from build123d import *

# Parameters (mm, degrees)
BASE_FLANGE1_START             = -11.5
BASE_FLANGE1_DEPTH             = 23
EDGE_FLANGE1_STRIP_W           = 7.0732
EDGE_FLANGE1_STRIP_H           = 1.4
EDGE_FLANGE1_STRIP_CUT_DEPTH   = 49.9268
EDGE_FLANGE1_STRIP_2_W         = 7.0732
EDGE_FLANGE1_STRIP_2_H         = 1.4
EDGE_FLANGE1_STRIP_CUT_2_DEPTH = 49.9268
EDGE_FLANGE1_DEPTH             = 49.9268
EDGE_FLANGE1_BEND_DEPTH        = 49.9268
FILLET1_RADIUS                 = 11.5
FILLET1_LENGTH                 = 1.4
FILLET2_RADIUS                 = 11.5
FILLET2_LENGTH                 = 1.4
SKETCH12_R                     = 4.05
SKETCH12_R_2                   = 0.9
CUT_EXTRUDE1_DEPTH             = 66.006845793
SKETCH13_R                     = 4.075
SKETCH13_R_2                   = 0.9
CUT_EXTRUDE2_DEPTH             = 45.973992485


# Read off the part's stored shape, not the designer's step: Base-Flange1
# Sheet-metal steps are written as plain solids
with BuildPart() as part:
    # Base-Flange1 outline → Base-Flange1 (new body)
    with BuildSketch(Plane(origin=(0, 0, 0), x_dir=(0, 0, -1), z_dir=(1, 0, 0)).offset(BASE_FLANGE1_START)):
        with BuildLine():
            Line((27.1, 2.1366), (27.1, 34))
            Line((27.1, 34), (25.7, 34))
            Line((25.7, 34), (25.7, 2.1366))
            ThreePointArc((25.7, 2.1366), (25.484254855, 1.615745145), (24.9634, 1.4))
            Line((24.9634, 1.4), (-24.9634, 1.4))
            ThreePointArc((-24.9634, 1.4), (-25.484254855, 1.615745145), (-25.7, 2.1366))
            Line((-25.7, 2.1366), (-25.7, 34))
            Line((-25.7, 34), (-27.1, 34))
            Line((-27.1, 34), (-27.1, 2.1366))
            ThreePointArc((-27.1, 2.1366), (-26.474204349, 0.625795651), (-24.9634, 0))
            Line((-24.9634, 0), (24.9634, 0))
            ThreePointArc((24.9634, 0), (26.474204349, 0.625795651), (27.1, 2.1366))
        make_face()
    extrude(amount=BASE_FLANGE1_DEPTH)

    # Edge-Flange1 strip (across the edge) → Edge-Flange1 strip cut (cut)
    with BuildSketch(Plane(origin=(11.5, 1.4, 24.9634), x_dir=(-1, 0, 0), z_dir=(0, 0, -1))):
        with Locations((-1.4, -0.7)):
            Rectangle(EDGE_FLANGE1_STRIP_W, EDGE_FLANGE1_STRIP_H)
    extrude(amount=EDGE_FLANGE1_STRIP_CUT_DEPTH, mode=Mode.SUBTRACT)

    # Edge-Flange1 strip 2 (across the edge) → Edge-Flange1 strip cut 2 (cut)
    with BuildSketch(Plane(origin=(-11.5, 1.4, -24.9634), x_dir=(1, 0, 0), z_dir=(0, 0, 1))):
        with Locations((-1.4, -0.7)):
            Rectangle(EDGE_FLANGE1_STRIP_2_W, EDGE_FLANGE1_STRIP_2_H)
    extrude(amount=EDGE_FLANGE1_STRIP_CUT_2_DEPTH, mode=Mode.SUBTRACT)

    # Edge-Flange1 section (across the edge) → Edge-Flange1 (add)
    with BuildSketch(Plane(origin=(11.5, 1.4, 24.9634), x_dir=(-1, 0, 0), z_dir=(0, 0, -1))):
        with BuildLine():
            Line((0, 0.7366), (0, 3.6))
            Line((0, 3.6), (1.4, 3.6))
            Line((1.4, 3.6), (1.4, 0.7366))
            ThreePointArc((1.4, 0.7366), (1.615745145, 0.215745145), (2.1366, 0))
            Line((2.1366, 0), (2.1366, -1.4))
            ThreePointArc((2.1366, -1.4), (0.625795651, -0.774204349), (0, 0.7366))
        make_face()
    extrude(amount=EDGE_FLANGE1_DEPTH)

    # Edge-Flange1 section 2 (across the edge) → Edge-Flange1 bend (add)
    with BuildSketch(Plane(origin=(-11.5, 1.4, -24.9634), x_dir=(1, 0, 0), z_dir=(0, 0, 1))):
        with BuildLine():
            Line((0, 0.7366), (0, 3.6))
            Line((0, 3.6), (1.4, 3.6))
            Line((1.4, 3.6), (1.4, 0.7366))
            ThreePointArc((1.4, 0.7366), (1.615745145, 0.215745145), (2.1366, 0))
            Line((2.1366, 0), (2.1366, -1.4))
            ThreePointArc((2.1366, -1.4), (0.625795651, -0.774204349), (0, 0.7366))
        make_face()
    extrude(amount=EDGE_FLANGE1_BEND_DEPTH)

    # Fillet1: full round fillet: the end face becomes a half cylinder, R = half its width
    fillet1_face = Plane((0, 34, 26.4), x_dir=(0, 0, 1), z_dir=(0, 1, 0))  # on the end face: x along it, z out of the body
    fillet1_slab = fillet1_face.offset(-FILLET1_RADIUS / 2) * Box(FILLET1_LENGTH, 2 * FILLET1_RADIUS, FILLET1_RADIUS, mode=Mode.PRIVATE)  # the body's end, R deep
    fillet1_round = Plane((0, 22.5, 26.4), x_dir=(0, 1, 0), z_dir=(0, 0, 1)) * Cylinder(FILLET1_RADIUS, FILLET1_LENGTH, mode=Mode.PRIVATE)  # its axis R under the face
    add(fillet1_slab - fillet1_round, mode=Mode.SUBTRACT)

    # Fillet2: full round fillet: the end face becomes a half cylinder, R = half its width
    fillet2_face = Plane((0, 34, -26.4), x_dir=(0, 0, 1), z_dir=(0, 1, 0))  # on the end face: x along it, z out of the body
    fillet2_slab = fillet2_face.offset(-FILLET2_RADIUS / 2) * Box(FILLET2_LENGTH, 2 * FILLET2_RADIUS, FILLET2_RADIUS, mode=Mode.PRIVATE)  # the body's end, R deep
    fillet2_round = Plane((0, 22.5, -26.4), x_dir=(0, 1, 0), z_dir=(0, 0, 1)) * Cylinder(FILLET2_RADIUS, FILLET2_LENGTH, mode=Mode.PRIVATE)  # its axis R under the face
    add(fillet2_slab - fillet2_round, mode=Mode.SUBTRACT)

    # Sketch12 → Cut-Extrude1 (cut, through all)
    with BuildSketch(Plane.XY.offset(27.1)):
        with Locations((0, 22.5)):
            Circle(SKETCH12_R)
        with Locations((0, 29.4)):
            Circle(SKETCH12_R_2)
        with Locations((6.9, 22.5)):
            Circle(SKETCH12_R_2)
        with Locations((0, 15.6)):
            Circle(SKETCH12_R_2)
        with Locations((-6.9, 22.5)):
            Circle(SKETCH12_R_2)
    extrude(amount=-CUT_EXTRUDE1_DEPTH, mode=Mode.SUBTRACT)

    # Sketch13 → Cut-Extrude2 (cut, through all)
    with BuildSketch(Plane(origin=(0, 0, 0), x_dir=(1, 0, 0), z_dir=(0, 1, 0))):
        with Locations(Location((0, 0, 0), (0, 0, 270))):
            Circle(SKETCH13_R)
        with Locations(Location((-4.87903679, 4.87903679, 0), (0, 0, 270))):
            Circle(SKETCH13_R_2)
        with Locations(Location((4.87903679, 4.87903679, 0), (0, 0, 270))):
            Circle(SKETCH13_R_2)
        with Locations(Location((4.87903679, -4.87903679, 0), (0, 0, 270))):
            Circle(SKETCH13_R_2)
        with Locations(Location((-4.87903679, -4.87903679, 0), (0, 0, 270))):
            Circle(SKETCH13_R_2)
        with Locations(Location((0, 13.35, 0), (0, 0, 270))):
            Circle(SKETCH13_R_2)
        with Locations(Location((0, -13.35, 0), (0, 0, 90))):
            Circle(SKETCH13_R_2)
    extrude(amount=CUT_EXTRUDE2_DEPTH, mode=Mode.SUBTRACT)


solid = part.part
Design review of the part built by this model. Coordinates are the model's own, in mm. A direction names the side the tool comes from. Coordinates: 2 decimals unless noted, no trailing zeros. Order: outer loops, then holes, each group sorted by start corner. A loop starts at its lowest first (then second) coordinate and runs counter-clockwise, first axis right, second up. Notation, with made-up numbers: (-7.75, 12.5) -> (50.25, 12.5) arc R30 cw to (50.25, 50.5) -> close; hole circle Ø5 at (53.5, 17.5). An arc over 180 degrees is marked (long way). One line per item, written item: value.
1) Draft analysis for pull direction X (two halves, no side actions). For faces 6 (the face through (0, 18, 27.1)), 7 (the face through (-0.12, 30.29, -26.39)), 8 (the face through (-0.12, 30.29, 26.41)), 9 (the face through (11.5, 11, -26)), state which applies: +X half, -X half, draft (parallel to the pull), parting line (faces both ways), or undercut.
Output values:
face 6: draft
face 7: undercut
face 8: undercut
face 9: +X half
2) Clearance check with flat-ended pins moving along their axes: P1, Ø2.5, axis at x = -4.88, z = 4.88, coming from the +Y side; P2, Ø1.6, axis at x = -6.9, y = 22.5, coming from the -Z side; P3, Ø1.1, axis at x = -10.5, y = 1, coming from the -Z side. State where each tip first meets the part, or that it passes through.
Output values:
P1: stops at y = 1.4
P2: passes through
P3: stops at z = -27.02
3) We need section A-A, the plane y = 12. Give the boundary of the cut face in (x, z).
Output values:
outline: (-11.5, -27.1) -> (11.5, -27.1) -> (11.5, -25.7) -> (-11.5, -25.7) -> close; (-11.5, 25.7) -> (11.5, 25.7) -> (11.5, 27.1) -> (-11.5, 27.1) -> close
4) To check wall thickness, follow probe 1 along Z at (x, y) = (6.75, 14.5); probe 2 along Y at (x, z) = (0, -26.05); probe 3 along Y at (x, z) = (0, 26.55). State the ranges of each line that lie inside material, in increasing order. Write a range as [from, to].
Output values:
probe 1: z = [-27.1, -25.7], [25.7, 27.1]
probe 2: y = [0.3, 14.7], [16.5, 18.45], [26.55, 28.5], [30.3, 34]
probe 3: y = [0.71, 14.7], [16.5, 18.45], [26.55, 28.5], [30.3, 34]
5) We need section C-C, the plane z = 0. Give the boundary of the cut face in (x, y) (3 decimals).
Output values:
outline: (-11.5, 2.137) arc R2.137 ccw to (-9.363, 0) -> (-4.075, 0) -> (-4.075, 1.4) -> (-9.363, 1.4) arc R0.737 cw to (-10.1, 2.137) -> (-10.1, 5) -> (-11.5, 5) -> close; (4.075, 0) -> (9.363, 0) arc R2.137 ccw to (11.5, 2.137) -> (11.5, 5) -> (10.1, 5) -> (10.1, 2.137) arc R0.737 cw to (9.363, 1.4) -> (4.075, 1.4) -> close
6) We need section B-B, the plane x = -6.9. Give the boundary of the cut face in (y, z).
Output values:
outline: (0, -24.96) arc R2.14 ccw to (2.14, -27.1) -> (21.6, -27.1) -> (21.6, -25.7) -> (2.14, -25.7) arc R0.74 cw to (1.4, -24.96) -> (1.4, 24.96) arc R0.74 cw to (2.14, 25.7) -> (21.6, 25.7) -> (21.6, 27.1) -> (2.14, 27.1) arc R2.14 ccw to (0, 24.96) -> close; (23.4, -27.1) -> (31.7, -27.1) -> (31.7, -25.7) -> (23.4, -25.7) -> close; (23.4, 25.7) -> (31.7, 25.7) -> (31.7, 27.1) -> (23.4, 27.1) -> close
7) We need section D-D, the plane y = 15.6. Give the boundary of the cut face in (x, z).
Output values:
outline: (-11.5, -27.1) -> (-0.9, -27.1) -> (-0.9, -25.7) -> (-11.5, -25.7) -> close; (-11.5, 25.7) -> (-0.9, 25.7) -> (-0.9, 27.1) -> (-11.5, 27.1) -> close; (0.9, -27.1) -> (11.5, -27.1) -> (11.5, -25.7) -> (0.9, -25.7) -> close; (0.9, 25.7) -> (11.5, 25.7) -> (11.5, 27.1) -> (0.9, 27.1) -> close
8) Machinability: for faces 1 (the face through (0, 18, -27.1)), 2 (the face through (-11, 0.4, 24.963)), 3 (the face through (-11.5, 11, -26)), 4 (the face through (10.86, 0.61, 0.35)), 5 (the face through (11, 5, 0)), which of the approach directions +Z, -Z, +X, -X, +Y, -Y give a long, thin tool a straight path to every point of the face, cutting with its end or side? Answer none if there is none.
Output values:
face 1: -Z, +X, -X, +Y, -Y
face 2: -X, -Y
face 3: +Z, -Z, -X, +Y, -Y
face 4: +X, -Y
face 5: +X, -X, +Y
